Source: CAD feature listing. Evaluate the final solid. Frame: model axes, mm. A direction names the side the tool comes from. Coordinates: 2 decimals unless noted, no trailing zeros. Order: outer loops, then holes, each group sorted by start corner. A loop starts at its lowest first (then second) coordinate and runs counter-clockwise, first axis right, second up. Notation, with made-up numbers: (44.5, 29.25) - (69.5, 29.25) arc R33 cw to (69.5, 67.25) - close; hole circle Ø5 at (2, 40.25). An arc over 180 degrees is marked (long way). One line per question, with ' | ' between items. Start each with the question number.
(1) Section C-C (y = 173.5). Return the cut outline in (x, z).
(2) Section A-A (x = 111.75). Return the cut outline in (y, z).
(3) Section B-B (z = 23). Return the cut outline in (x, y).
(4) Line query: line 1 along Z through (x, y) = (117.5, 179.04); line 2 along Z through (x, y) = (118.7, 179.04); line 3 along X through (y, z) = (123.5, 65.7). Output: solid intervals per line, ascending.
(5) Access query for faces 1 (the cylindrical face through (118.71, 192.89, 13.35)), 2 (the cylindrical face through (101.64, 172.03, 65.79)), 3 (the flat face through (110, 132.5, 66)). Directions: +Z, -Z, +X, -X, +Y, -Y. A direction counts if a zero-diameter tool reaches every point of the face in a straight line with its end or side. Return the directions, or none.
(6) Section D-D (z = 45.22). Return the cut outline in (x, y).
(7) Draft query along Y for faces 4 (the cylindrical face through (118.712, 112.617, 59.463)), 5 (the flat face through (119, 206, 50)), 6 (the flat face through (110, 182.5, 66)), 7 (the flat face through (105.15, 173.57, 68.5)). Return one class per face: +Y half, -Y half, draft (parallel to the pull), parting line (faces both ways), or undercut.
(8) Contact query for flat-ended pins moving along their axis: P1, Ø4.5, axis at x = 102.99, y = 173.5, coming from the +Z side; P2, Ø3.5, axis at x = 119.5, y = 90.5, coming from the +Z side; P3, Ø3.5, axis at y = 179.04, z = 17.28, coming from the +X side; P4, Ø3, axis at x = 109.5, z = 66.5, coming from the -Y side. Output: stop coordinate, or through.
Solid Edge part; units mm, degrees
extrude "Protrusion1" [suppressed]
sketch "Sketch1" plane through (116.4938, 148.5, 37.25) normal (1, 0, 0) x (0, 1, 0)
  line L0 (72.5, -6.75) -> (72.5, 12.75)
  line L1 (72.5, 12.75) -> (41.5, 12.75)
  arc A0 (34, 32.75) -> (41.5, 12.75) centre (64.4167, 32.75) ccw
  line L2 (0, 32.75) -> (34, 32.75)
  line L3 (0, 32.75) -> (-34, 32.75)
  arc A1 (-34, 32.75) -> (-41.5, 12.75) centre (-64.4167, 32.75) cw
  line L4 (-41.5, 12.75) -> (-72.5, 12.75)
  line L5 (-72.5, -6.75) -> (-72.5, 12.75)
  arc A2 (-72.5, -21.75) -> (-72.5, -6.75) centre (-72.5, -14.25) cw
  line L6 (-72.5, -32.25) -> (-72.5, -21.75)
  line L7 (72.5, -32.25) -> (-72.5, -32.25)
  line L8 (72.5, -21.75) -> (72.5, -32.25)
  arc A3 (72.5, -21.75) -> (72.5, -6.75) centre (72.5, -14.25) ccw
  circle A4 centre (72.5, -14.25) radius 2
  circle A5 centre (-72.5, -14.25) radius 2
  circle A6 centre (-20.26, 23.21) radius 1.6
  circle A7 centre (30.54, 7.97) radius 1.6
  circle A8 centre (30.54, -19.97) radius 1.6
  line L9 (66.3808, -16.75) -> (66.3808, -11.75)
  arc A9 (56.3808, -1.75) -> (66.3808, -11.75) centre (56.3808, -11.75) cw
  line L10 (56.3808, -1.75) -> (51.3808, -1.75)
  arc A10 (41.3808, -11.75) -> (51.3808, -1.75) centre (51.3808, -11.75) cw
  line L11 (41.3808, -11.75) -> (41.3808, -16.75)
  arc A11 (41.3808, -16.75) -> (51.3808, -26.75) centre (51.3808, -16.75) ccw
  line L12 (51.3808, -26.75) -> (56.3808, -26.75)
  arc A12 (66.3808, -16.75) -> (56.3808, -26.75) centre (56.3808, -16.75) cw
extrude "Protrusion2" add sketch "Sketch1" along normal blind 4.5
sketch "Sketch2" plane through (106.8492, 148.5, 70) normal (0, 0, 1) x (0, 1, 0)
  circle A0 centre (-25, 3.8554) radius 2
  line L0 (-16, 3.8554) -> (-16, -9.6446)
  line L1 (-34, -9.6446) -> (-16, -9.6446)
  line L2 (-34, 3.8554) -> (-34, -9.6446)
  arc A1 (-34, 3.8554) -> (-16, 3.8554) centre (-25, 3.8554) cw
  circle A2 centre (25, 3.8554) radius 2
  line L3 (16, 3.8554) -> (16, -9.6446)
  line L4 (16, -9.6446) -> (34, -9.6446)
  line L5 (34, 3.8554) -> (34, -9.6446)
  arc A3 (34, 3.8554) -> (16, 3.8554) centre (25, 3.8554) ccw
extrude "ProtrusiónExtruida_24" add sketch "Sketch2" against normal blind 7
fillet "Redondeo_4" radius 3 5 edges at (116.4938, 173.5, 63) (116.4938, 123.5, 63) (116.4938, 173.5, 63) (116.4938, 123.5, 63) (120.9938, 148.5, 70)
fillet "Redondeo_5" [suppressed]
sketch "Sketch3" plane through (108.6188, 148.5, 70) normal (0, 0, 1) x (0, 1, 0)
  circle A0 centre (-25, 5.625) radius 5
  circle A1 centre (25, 5.625) radius 5
extrude "VaciadoExtruido_57" cut sketch "Sketch3" along normal mid plane 3
Response values:
1) outline: (93.99, 63) - (100.99, 63) - (100.99, 68.5) - (97.99, 68.5) - (97.99, 70) - (93.99, 70) - close; (104.99, 63) - (113.49, 63) arc R3 cw to (116.49, 60) - (116.49, 5) - (120.99, 5) - (120.99, 67) arc R3 ccw to (117.99, 70) - (107.99, 70) - (107.99, 68.5) - (104.99, 68.5) - close
2) outline: (114.5, 63) - (132.5, 63) - (132.5, 70) - (114.5, 70) - close; (164.5, 63) - (182.5, 63) - (182.5, 70) - (164.5, 70) - close
3) outline: (116.49, 68.5) - (120.99, 68.5) - (120.99, 74) - (116.49, 74) - close; (116.49, 78) - (120.99, 78) - (120.99, 189.88) - (116.49, 189.88) - close; (116.49, 214.88) - (120.99, 214.88) - (120.99, 219) - (116.49, 219) - close; (116.49, 223) - (120.99, 223) - (120.99, 228.5) - (116.49, 228.5) - close
4) line 1: z = 5 to 15.68, 18.88 to 43.62, 46.82 to 70 | line 2: z = 5 to 15.68, 18.88 to 43.62, 46.82 to 69.92 | line 3: x = 93.99 to 100.99, 104.99 to 120.99
5) face 1: +X, -X | face 2: +Z, -Z | face 3: +Z, -Z, -X
6) outline: (116.49, 76) - (120.99, 76) - (120.99, 177.44) - (116.49, 177.44) - close; (116.49, 180.64) - (120.99, 180.64) - (120.99, 221) - (116.49, 221) - close
7) face 4: -Y half | face 5: draft | face 6: +Y half | face 7: undercut
8) P1: stops at z = 68.5 | P2: stops at z = 50 | P3: stops at x = 120.99 | P4: stops at y = 114.5
